Part model, mm, in its own coordinate system. A direction names the side the tool comes from. Round coordinates to 2 decimals unless told otherwise and drop trailing zeros. Loops run counter-clockwise (first coordinate to the right, second up) from the corner with the lowest first, then second, coordinate; pieces in that order, holes last. Notation, with made-up numbers: (-21.75, 25) -> (0.25, 25) arc R24 ccw to (0.25, 46) -> close; hole circle Ø2 at (36.5, 54). An arc over 180 degrees is marked (long way). Answer as a JSON object with one key per item and string values. Group by question number.
Autodesk Inventor part; units mm, degrees
ref_plane "YZ Plane" through (0, 0, 0) normal (1, 0, 0) x (0, 1, 0)
ref_plane "XZ Plane" through (0, 0, 0) normal (0, 1, 0) x (-1, 0, 0)
ref_plane "XY Plane" through (0, 0, 0) normal (0, 0, 1) x (1, 0, 0)
sketch "Sketch1" plane through (0, 0, 0) normal (0, 0, 1) x (1, 0, 0)
  circle A0 centre (0, 0) radius 25.4
  dimension "d0" = 50.8
extrude "Extrusion1" add sketch "Sketch1" along normal blind 12.7
sketch "Sketch2" plane through (0, 0, 12.7) normal (0, 0, 1) x (1, 0, 0)
  line L0 (0, 3.1852) -> (2.7584, 1.5926)
  line L1 (2.7584, 1.5926) -> (2.7584, -1.5926)
  line L2 (2.7584, -1.5926) -> (0, -3.1852)
  line L3 (0, -3.1852) -> (-2.7584, -1.5926)
  line L4 (-2.7584, -1.5926) -> (-2.7584, 1.5926)
  line L5 (-2.7584, 1.5926) -> (0, 3.1852)
  point P0 (0, 0)
  point P1 (0, 0)
  dimension "d3" = 3.1852
extrude "Extrusion2" cut sketch "Sketch2" against normal through all
sketch "Sketch3" plane through (0, 0, 12.7) normal (0, 0, 1) x (1, 0, 0)
  circle A0 centre (0, 0) radius 9.525
  dimension "d6" = 19.05
extrude "Extrusion3" cut sketch "Sketch3" against normal blind 3.175
fillet "Fillet3" radius 1.27 4 edges at (-25.4, 0, 12.7) (-25.4, 0, 0) (-9.525, 0, 12.7) (-9.525, 0, 9.525)
properties part number "BallShooterWheel000105"
Item 1: Drill centre lines: line 1 (Y direction, x = 0, z = 11.35) (3 decimals); line 2 (Y direction, x = -2.5, z = 3); line 3 (Z direction, x = -0.5, y = -6.5) (3 decimals). Where is each one in solid material? Low to high.
Item 2: Band-saw the part on B-B, the plane z = 6.5. List the corners of the cut face in (x, y).
Item 3: Band-saw the part on A-A, the plane y = 0. List the corners of the cut face in (x, z) (3 decimals), plus the area to 3 significant figures.
Item 4: Which spindle directions (+Z, -Z, +X, -X, +Y, -Y) get a long thin tool onto all of the face, cutting with end or side? Do faces 1 (the face through (10, -5, 12.7)), 2 (the face through (1.399, -2.378, 4.829)), 3 (the face through (-7.559, -5.796, 11.117)). Say none if no direction does.
Item 5: Two-plate mould, pull along X, no slides. Class faces 4 (the face through (-1.36, -2.4, 4.83)), 5 (the face through (-5.506, 24.796, 6.279)), 6 (the face through (0, -5, 0)): pulls with the +X half, pulls with the -X half, needs draft (parallel to the pull), parting line crosses it, or undercut.
Item 6: Drop flat-ended pins along their axis: pin 1 Ø1 at (y, z) = (5, 8) entering from +X; pin 2 Ø2 at (y, z) = (-16, 5.5) entering from -X; pin 3 Ø6 at (x, z) = (18, 4.5) entering from -Y. Give the stop position or say it passes through.
Entries:
{
 "1": {"line 1": "-25.4 to -9.525, 9.525 to 25.4", "line 2": "-25.28 to -1.74, 1.74 to 25.28", "line 3": "0 to 9.525"},
 "2": {"outline": "circle Ø50.8 at (0, 0); hole (-2.76, -1.59) -> (0, -3.19) -> (2.76, -1.59) -> (2.76, 1.59) -> (0, 3.19) -> (-2.76, 1.59) -> close"},
 "3": {"outline": "(-25.4, 1.27) arc R1.27 ccw to (-24.13, 0) -> (-2.758, 0) -> (-2.758, 9.525) -> (-8.255, 9.525) arc R1.27 cw to (-9.525, 10.795) -> (-9.525, 11.43) arc R1.27 ccw to (-10.795, 12.7) -> (-24.13, 12.7) arc R1.27 ccw to (-25.4, 11.43) -> close; (2.758, 0) -> (24.13, 0) arc R1.27 ccw to (25.4, 1.27) -> (25.4, 11.43) arc R1.27 ccw to (24.13, 12.7) -> (10.795, 12.7) arc R1.27 ccw to (9.525, 11.43) -> (9.525, 10.795) arc R1.27 cw to (8.255, 9.525) -> (2.758, 9.525) -> close", "area": "531 mm²"},
 "4": {"face 1": "+Z, +X, -X, +Y, -Y", "face 2": "+Z, -Z", "face 3": "+Z"},
 "5": {"face 4": "undercut", "face 5": "parting line crosses it", "face 6": "needs draft"},
 "6": {"pin 1": "x = 25", "pin 2": "x = -20.5", "pin 3": "y = -20.5"}
}
